Source: CAD feature listing. Evaluate the final solid. Frame: model axes, mm. Round coordinates to 2 decimals unless told otherwise and drop trailing zeros. Write each loop counter-clockwise with the first axis right and the second up, starting at its lowest first coordinate (ties: lowest second). Pieces come first, ordered by that corner, then holes. Notation, with made-up numbers: M -1.75,36.25 L 57.25,36.25 A19 cw 57.25,55.25 Z; hole C 4.5,58.25 d2. An arc over 180 degrees is marked long. Answer in a Markdown table with one row per item.
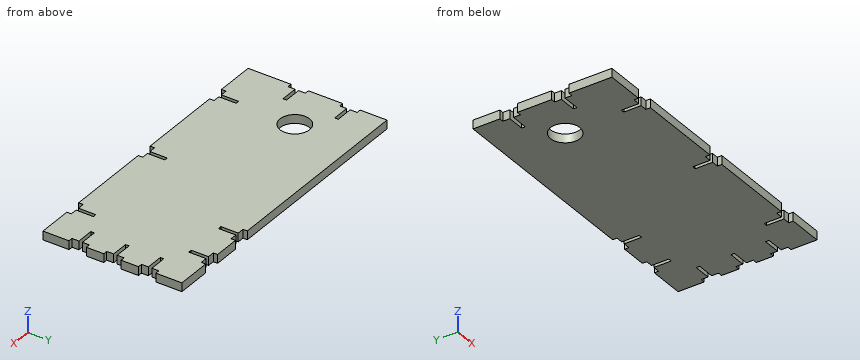
from build123d import *

# Parameters (mm, degrees)
BOSS_EXTRUDE1_DEPTH     = 6.35
CUT_EXTRUDE4_DEPTH      = 127
CUT_EXTRUDE4_DEPTH_BACK = 127
CUT_EXTRUDE5_DEPTH      = 127
CUT_EXTRUDE5_DEPTH_BACK = 127
SKETCH5_W               = 229.808362084
SKETCH5_H               = 77.917038349
CUT_EXTRUDE7_DEPTH      = 127
CUT_EXTRUDE7_DEPTH_BACK = 127
SKETCH6_R               = 10.795
CUT_EXTRUDE8_DEPTH      = 127
CUT_EXTRUDE8_DEPTH_BACK = 127


with BuildPart() as part:
    # Sketch1 → Boss-Extrude1 (new body)
    with BuildSketch(Plane.XY):
        Polygon((0, 0), (127, 0), (127, 101.6), (0, 101.6), (-70.692427737, 172.292427737), (-91.896861793, 151.087993682), (-91.896861793, 0), align=None)
    extrude(amount=BOSS_EXTRUDE1_DEPTH)

    # Sketch3 → Cut-Extrude4 (cut, two sides)
    with BuildSketch(Plane(origin=(0, 0, 0), x_dir=(-1, 0, 0), z_dir=(0, 0, -1))) as cut_extrude4_sk:
        Polygon((-88.9, 101.6), (-101.6, 101.6), (-101.6, 98.425), (-96.5327, 98.425), (-96.5327, 85.725), (-93.9673, 85.725), (-93.9673, 98.425), (-88.9, 98.425), align=None)
        Polygon((-57.15, 101.6), (-69.85, 101.6), (-69.85, 98.425), (-64.77, 98.425), (-64.77, 85.725), (-62.23, 85.725), (-62.23, 98.425), (-57.15, 98.425), align=None)
        Polygon((-127, 82.55), (-127, 69.85), (-123.825, 69.85), (-123.825, 74.9173), (-111.125, 74.9173), (-111.125, 77.4827), (-123.825, 77.4827), (-123.825, 82.55), align=None)
        Polygon((-127, 57.15), (-127, 44.45), (-123.825, 44.45), (-123.825, 49.5173), (-111.125, 49.5173), (-111.125, 52.0827), (-123.825, 52.0827), (-123.825, 57.15), align=None)
        Polygon((-127, 31.75), (-127, 25.4), (-127, 19.05), (-123.825, 19.05), (-123.825, 24.1173), (-111.125, 24.1173), (-111.125, 26.6827), (-123.825, 26.6827), (-123.825, 31.75), align=None)
        Polygon((-101.6, 3.302), (-101.6, 0), (-88.9, 0), (-88.9, 3.302), (-93.9673, 3.302), (-93.9673, 16.002), (-96.5327, 16.002), (-96.5327, 3.302), align=None)
        Polygon((-25.4, 3.302), (-25.4, 0), (-12.7, 0), (-12.7, 3.302), (-17.7673, 3.302), (-17.7673, 16.002), (-20.3327, 16.002), (-20.3327, 3.302), align=None)
        Polygon((50.8, 3.302), (50.8, 0), (63.5, 0), (63.5, 3.302), (58.4327, 3.302), (58.4327, 16.002), (55.8673, 16.002), (55.8673, 3.302), align=None)
        Polygon((88.721861793, 31.42199842), (91.896861793, 31.42199842), (91.896861793, 44.12199842), (88.721861793, 44.12199842), (88.721861793, 39.05469842), (76.021861793, 39.05469842), (76.021861793, 36.48929842), (88.721861793, 36.48929842), align=None)
        Polygon((88.721861793, 69.193996841), (91.896861793, 69.193996841), (91.896861793, 81.893996841), (88.721861793, 81.893996841), (88.721861793, 76.826696841), (76.021861793, 76.826696841), (76.021861793, 74.261296841), (88.721861793, 74.261296841), align=None)
        Polygon((88.721861793, 106.965995261), (91.896861793, 106.965995261), (91.896861793, 119.665995261), (88.721861793, 119.665995261), (88.721861793, 114.598695261), (76.021861793, 114.598695261), (76.021861793, 112.033295261), (88.721861793, 112.033295261), align=None)
        Polygon((70.692427737, 158.822043556), (66.202299677, 154.331915495), (63.957235647, 156.576979525), (68.447363707, 161.067107586), align=None)
    extrude(amount=CUT_EXTRUDE4_DEPTH, mode=Mode.SUBTRACT)
    extrude(cut_extrude4_sk.sketch, amount=-CUT_EXTRUDE4_DEPTH_BACK, mode=Mode.SUBTRACT)

    # Sketch4 → Cut-Extrude5 (cut, two sides)
    with BuildSketch(Plane.XY) as cut_extrude5_sk:
        Polygon((-81.917747889, 147.596723404), (-79.672683858, 149.841787435), (-75.182555798, 145.351659374), (-77.427619828, 143.106595344), align=None)
    extrude(amount=CUT_EXTRUDE5_DEPTH, mode=Mode.SUBTRACT)
    extrude(cut_extrude5_sk.sketch, amount=-CUT_EXTRUDE5_DEPTH_BACK, mode=Mode.SUBTRACT)

    # Sketch5 → Cut-Extrude7 (cut, two sides)
    with BuildSketch(Plane.XY) as cut_extrude7_sk:
        with Locations((12.095818958, 140.558519175)):
            Rectangle(SKETCH5_W, SKETCH5_H)
    extrude(amount=CUT_EXTRUDE7_DEPTH, mode=Mode.SUBTRACT)
    extrude(cut_extrude7_sk.sketch, amount=-CUT_EXTRUDE7_DEPTH_BACK, mode=Mode.SUBTRACT)

    # Sketch6 → Cut-Extrude8 (cut, two sides)
    with BuildSketch(Plane(origin=(0, 0, -2.54), x_dir=(-1, 0, 0), z_dir=(0, 0, -1))) as cut_extrude8_sk:
        with Locations((56.601909208, 58.354277065)):
            Circle(SKETCH6_R)
    extrude(amount=CUT_EXTRUDE8_DEPTH, mode=Mode.SUBTRACT)
    extrude(cut_extrude8_sk.sketch, amount=-CUT_EXTRUDE8_DEPTH_BACK, mode=Mode.SUBTRACT)


solid = part.part
Q1. Material intervals for probe 1 along X at (y, z) = (89, 3); probe 2 along Y at (x, z) = (112, 0.5); probe 3 along X at (y, z) = (13, 5.5), sorted ascending.
Solutions:
| item | result |
|---|---|
| probe 1 | x = -91.9 to 62.23, 64.77 to 93.97, 96.53 to 127 |
| probe 2 | y = 0 to 24.12, 26.68 to 49.52, 52.08 to 74.92, 77.48 to 101.6 |
| probe 3 | x = -91.9 to -58.43, -55.87 to 17.77, 20.33 to 93.97, 96.53 to 127 |
Q2. Section B-B (y = 11). Return loops of the section in (x, z).
Solutions:
| item | result |
|---|---|
| outline | M -91.9,0 L -58.43,0 L -58.43,6.35 L -91.9,6.35 Z; M -55.87,0 L 17.77,0 L 17.77,6.35 L -55.87,6.35 Z; M 20.33,0 L 93.97,0 L 93.97,6.35 L 20.33,6.35 Z; M 96.53,0 L 127,0 L 127,6.35 L 96.53,6.35 Z |
Q3. Contact query for flat-ended pins moving along their axis: pin 1 Ø2 at (y, z) = (77, 5.5) entering from -X; pin 2 Ø2.5 at (x, z) = (68, 4) entering from +Y (3 decimals); pin 3 Ø1.3 at (x, z) = (-57.5, 2.5) entering from -Y. Output: stop coordinate, or through.
Solutions:
| item | result |
|---|---|
| pin 1 | stops at x = -88.72 |
| pin 2 | stops at y = 98.425 |
| pin 3 | stops at y = 16 |
Q4. Section A-A (y = 89). Return loops of the section in (x, z), and give its area (3 significant figures).
Solutions:
| item | result |
|---|---|
| outline | M -91.9,0 L 62.23,0 L 62.23,6.35 L -91.9,6.35 Z; M 64.77,0 L 93.97,0 L 93.97,6.35 L 64.77,6.35 Z; M 96.53,0 L 127,0 L 127,6.35 L 96.53,6.35 Z |
| area | 1,360 mm2 |
Q5. Section C-C (y = 55). Return loops of the section in (x, z) (3 decimals).
Solutions:
| item | result |
|---|---|
| outline | M -91.897,0 L -66.863,0 L -66.863,6.35 L -91.897,6.35 Z; M -46.341,0 L 123.825,0 L 123.825,6.35 L -46.341,6.35 Z |
